Verification items for the finished model (mm, model axes). Round coordinates to 2 decimals unless told otherwise and drop trailing zeros. Write each loop counter-clockwise with the first axis right and the second up, starting at its lowest first coordinate (ties: lowest second). Pieces come first, ordered by that corner, then holes. Notation, with made-up numbers: (67.25, -17) - (114.25, -17) arc R8 ccw to (114.25, -13) - close; hole circle Ø10 at (86.25, -25.75). An arc over 180 degrees is marked (long way). Write each question's results on one line, items separated by ' | '.
```python
from build123d import *

# Parameters (mm, degrees)
F0_W     = 48
F0_H     = 48
F1_DEPTH = 24
F2_R     = 9
F3_DEPTH = 48
F5_DEPTH = 48


with BuildPart() as f1:
    # F0 (on Front) → F1 (new body, symmetric)
    with BuildSketch(Plane.XZ):
        Rectangle(F0_W, F0_H)
    extrude(amount=F1_DEPTH, both=True)

    # F2 (on face) → F3 (cut)
    with BuildSketch(Plane.XZ.offset(24)):
        with Locations((0, 24)):
            Circle(F2_R)
    extrude(amount=-F3_DEPTH, mode=Mode.SUBTRACT)

    # F4 (on face) → F5 (cut)
    with BuildSketch(Plane.YZ.offset(24)):
        with BuildLine():
            ThreePointArc((-9, 24), (0, 15), (9, 24))
            Line((9, 24), (-9, 24))
        make_face()
    extrude(amount=-F5_DEPTH, mode=Mode.SUBTRACT)


solid = f1.part
```
(1) Mould release check, pull along X, two halves, no side actions. Record for faces 1 (the flat face through (0, 24, 0)), 2 (the cylindrical face through (0, 14, 15)), 3 (the flat face through (-24, 0, 0)): released by +X, released by -X, zero draft, split by the parting line, or undercut.
Answer:
face 1: zero draft | face 2: undercut | face 3: released by -X
(2) Thickness scan on L1, parallel to Z at x = -1, y = -18; L2, parallel to Z at x = 4, y = -13. Record the ranges inside material, lowest first.
Answer:
L1: -24 to 15.06 | L2: -24 to 15.94
(3) Section check A-A (y = 18). Record the cut outline in (x, z), plus the area to 3 significant figures.
Answer:
outline: (-24, -24) - (24, -24) - (24, 24) - (9, 24) arc R9 cw to (-9, 24) - (-24, 24) - close | area: 2,180 mm2
(4) Go/stop test with a flat-tipped pin: pin 1 Ø3 at (x, y) = (1, -15) entering from +Z. Record where the tip stops, or that it passes through.
Answer:
pin 1: z = 15.35
